```python
from build123d import *

# Parameters (mm, degrees)
SKETCH1_R           = 25.4
BOSS_EXTRUDE1_DEPTH = 2.54
SKETCH2_R           = 6.35
BOSS_EXTRUDE2_DEPTH = 381


with BuildPart() as part:
    # Sketch1 → Boss-Extrude1 (new body)
    with BuildSketch(Plane(origin=(0, 0, 0), x_dir=(1, 0, 0), z_dir=(0, 1, 0))):
        with Locations(Location((0, 0, 0), (0, 0, 270))):
            Circle(SKETCH1_R)
    extrude(amount=BOSS_EXTRUDE1_DEPTH)

    # Sketch2 → Boss-Extrude2 (add)
    with BuildSketch(Plane(origin=(0, 2.54, 0), x_dir=(1, 0, 0), z_dir=(0, 1, 0))):
        with Locations(Location((0, 0, 0), (0, 0, 270))):
            Circle(SKETCH2_R)
    extrude(amount=-BOSS_EXTRUDE2_DEPTH)

    # Loft1: read off the stored shape, not the designer's step
    # Loft1: loft between two sections, ruled curve by curve
    loft1_from = [
        Edge.make_bspline([(4.913042865, -378.46, -4.022997615), (12.959038094, -378.46, 5.803088115), (3.132952365, -378.46, 13.849083344), (-4.913042865, -378.46, 4.022997615), (-12.959038094, -378.46, -5.803088115), (-3.132952365, -378.46, -13.849083344), (4.913042865, -378.46, -4.022997615)], [0, 0, 0, 0, 0.5, 0.5, 0.5, 1, 1, 1, 1], 3, [1, 0.333333333, 0.333333333, 1, 0.333333333, 0.333333333, 1]),
    ]
    loft1_to = [
        Edge.make_bspline([(-0.252067696, -406.4, -1.244733657), (2.237399617, -406.4, -1.748869049), (2.74153501, -406.4, 0.740598264), (0.252067696, -406.4, 1.244733657), (-2.237399617, -406.4, 1.748869049), (-2.74153501, -406.4, -0.740598264), (-0.252067696, -406.4, -1.244733657)], [0, 0, 0, 0, 0.5, 0.5, 0.5, 1, 1, 1, 1], 3, [1, 0.333333333, 0.333333333, 1, 0.333333333, 0.333333333, 1]),
    ]
    loft1 = Solid(Shell([*[Face.make_surface_from_curves(loft1_from[k], loft1_to[k]) for k in range(1)], Face(Wire(loft1_from)), Face(Wire(loft1_to))]))
    add(loft1)


solid = part.part
```
Source: CAD feature listing. Evaluate the final solid. Frame: model axes, mm. A direction names the side the tool comes from. Coordinates: 2 decimals unless noted, no trailing zeros. Loops run counter-clockwise (first coordinate to the right, second up) from the corner with the lowest first, then second, coordinate; pieces in that order, holes last. Notation, with made-up numbers: M 37,50 L 88,50 A19 cw 88,75 Z; hole C 65.25,60 d9. An arc over 180 degrees is marked long. Use a Markdown table: item, result. Add a question column.
Q1. Section query B-B, the plane x = 10.5. Return loops of the section in (y, z), and give its area (3 significant figures).
Q2. Section query A-A, the plane y = -120. Return loops of the section in (x, z).
Q3. First-contact query: pin 1 (1 mm diameter, centred on x = -18, z = -5.5, fed in from -Y); pin 2 (6 mm diameter, centred on x = -12, y = -176, fed in from +Z). Flat tips, straight axial feed; report the tip coordinate or a pass-through.
Q4. Access query for faces 1 (the flat face through (-5, 0, 5)), 2 (the flat face through (0, 2.54, 0)). Directions: +Z, -Z, +X, -X, +Y, -Y. A direction counts if a zero-diameter tool reaches every point of the face in a straight line with its end or side. Return the directions, or none.
Q5. Section query C-C, the plane x = -16. Return loops of the section in (y, z), and give its area (3 significant figures).
Q6. Material intervals for L1, parallel to Y at x = -3, z = 13; L2, parallel to X at y = -26, z = 1; L3, parallel to X at y = -54, z = 2, sorted ascending.
Result:
| question | item | result |
|---|---|---|
| 1 | outline | M 0,-23.13 L 2.54,-23.13 L 2.54,23.13 L 0,23.13 Z |
| 1 | area | 117 mm2 |
| 2 | outline | C 0,0 d12.7 |
| 3 | pin 1 | stops at y = 0 |
| 3 | pin 2 | passes through |
| 4 | face 1 | -Y |
| 4 | face 2 | +Z, -Z, +X, -X, +Y |
| 5 | outline | M 0,-19.73 L 2.54,-19.73 L 2.54,19.73 L 0,19.73 Z |
| 5 | area | 100 mm2 |
| 6 | L1 | y = 0 to 2.54 |
| 6 | L2 | x = -6.27 to 6.27 |
| 6 | L3 | x = -6.03 to 6.03 |
